For this review, take the finished solid that the model builds, in its own axes (mm). Face numbers are marked on the shaded views. Coordinates: 2 decimals unless noted, no trailing zeros. Loops run counter-clockwise (first coordinate to the right, second up) from the corner with the lowest first, then second, coordinate; pieces in that order, holes last. Notation, with made-up numbers: (54.5, 2.25) - (78.5, 2.25) arc R23 cw to (78.5, 27.25) - close; hole circle Ø8 at (82, -2). An arc over 180 degrees is marked (long way). Answer as a JSON object with one key per item and string values. Group by question number.
Item 1: We need section A-A (z = 5.25). Give the boundary of the cut face in (x, y).
Item 2: Mouldability with a two-part tool opening along X and no side actions: class the marked faces 1, 2 and 3 as released by +X, released by -X, zero draft, split by the parting line, or undercut.
Item 3: We need section C-C (y = -48). Give the boundary of the cut face in (x, z), then the cut area to 3 significant figures.
Item 4: We need section B-B (x = -4.85). Give the boundary of the cut face in (y, z).
Item 5: We need section D-D (z = 4.1). Give the boundary of the cut face in (x, y), then the cut area to 3 significant figures.
Item 6: To check wall thickness, follow line 1 (Y direction, x = -4.85, z = 3.2); line 2 (X direction, y = -56.25, z = 3.8); line 3 (X direction, y = -56.75, z = 3.3). State the ranges of each line that lie inside material, in increasing order.
Item 7: Clearance check with flat-ended pins moving along their axes: pin 1 (2 mm diameter, centred on y = -53, z = 4, fed in from +X); pin 2 (1.5 mm diameter, centred on y = -53.5, z = 4, fed in from -X). State where each tip first meets the part, or that it passes through.
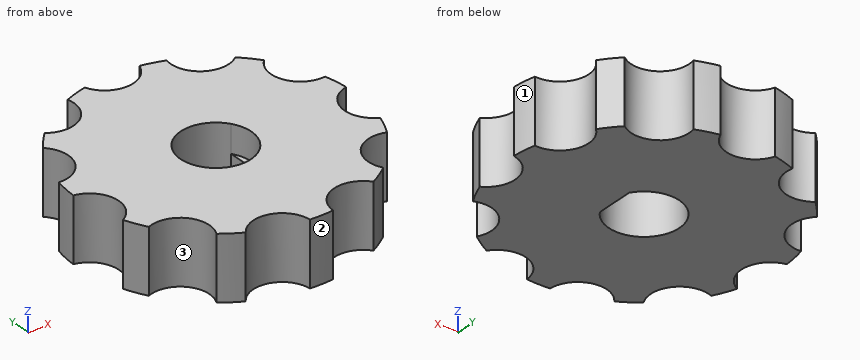
from build123d import *

# Parameters (mm, degrees)
SKETCH024_R           = 9.9166910254
PAD016_DEPTH          = 4.6
SKETCH025_R           = 2.1
POCKET004_DEPTH       = 61.4476740325
POLARPATTERN001_COUNT = 11
POCKET005_DEPTH       = 4.601
SKETCH037_R           = 2.55
POCKET012_DEPTH       = 2


with BuildPart() as part:
    # Sketch024 → Pad016 (new body)
    with BuildSketch(Plane.XY):
        Circle(SKETCH024_R)
    extrude(amount=PAD016_DEPTH)

    # Sketch025 (on Face3 of Pad016) → Pocket004 (cut, through all)
    with BuildSketch(Plane.XY.offset(4.6)):
        with Locations((0, 10.4166910254)):
            Circle(SKETCH025_R)
    pocket004 = extrude(amount=-POCKET004_DEPTH, mode=Mode.SUBTRACT)

    # PolarPattern001: Pocket004 ×11 about axis
    polarpattern001_axis = Axis((0, 0, 4.6), (0, 0, 1))
    for i in range(1, POLARPATTERN001_COUNT):
        add(pocket004.rotate(polarpattern001_axis, i * 360 / POLARPATTERN001_COUNT), mode=Mode.SUBTRACT)

    # Sketch026 (on Face4 of PolarPattern001) → Pocket005 (cut, through all)
    with BuildSketch(Plane.XY.offset(4.6)):
        with BuildLine():
            ThreePointArc((2.15, 1.3711309201), (-2.55, 0), (2.15, -1.3711309201))
            Line((2.15, -1.3711309201), (2.15, 1.3711309201))
        make_face()
    extrude(amount=-POCKET005_DEPTH, mode=Mode.SUBTRACT)

    # Sketch037 (on Face4 of Pocket005) → Pocket012 (cut)
    with BuildSketch(Plane.XY.offset(4.6)):
        Circle(SKETCH037_R)
    extrude(amount=-POCKET012_DEPTH, mode=Mode.SUBTRACT)


with BuildPart() as part_1:
    # Body004 placement: moved
    add(part.part.moved(Location((-4.85, -48.15, 2.2))))


solid = part_1.part
Check sheet entries:
{
 "1": {"outline": "(-14.75, -47.57) arc R2.1 cw to (-14.19, -51.49) arc R9.92 ccw to (-13.49, -53.02) arc R2.1 cw to (-10.9, -56.01) arc R9.92 ccw to (-9.49, -56.92) arc R2.1 cw to (-5.69, -58.03) arc R9.92 ccw to (-4.01, -58.03) arc R2.1 cw to (-0.21, -56.92) arc R9.92 ccw to (1.2, -56.01) arc R2.1 cw to (3.79, -53.02) arc R9.92 ccw to (4.49, -51.49) arc R2.1 cw to (5.05, -47.57) arc R9.92 ccw to (4.81, -45.91) arc R2.1 cw to (3.17, -42.31) arc R9.92 ccw to (2.07, -41.05) arc R2.1 cw to (-1.26, -38.91) arc R9.92 ccw to (-2.87, -38.43) arc R2.1 cw to (-6.83, -38.43) arc R9.92 ccw to (-8.44, -38.91) arc R2.1 cw to (-11.77, -41.05) arc R9.92 ccw to (-12.87, -42.31) arc R2.1 cw to (-14.51, -45.91) arc R9.92 ccw to start; hole circle Ø5.1 at (-4.85, -48.15)"},
 "2": {"face 1": "released by +X", "face 2": "split by the parting line", "face 3": "undercut"},
 "3": {"outline": "(-13.84, 2.2) - (-7.4, 2.2) - (-7.4, 6.8) - (-13.84, 6.8) - close; (-2.7, 2.2) - (4.14, 2.2) - (4.14, 6.8) - (-2.3, 6.8) - (-2.3, 4.8) - (-2.7, 4.8) - close", "area": "60.3 mm2"},
 "4": {"outline": "(-58.07, 2.2) - (-50.7, 2.2) - (-50.7, 6.8) - (-58.07, 6.8) - close; (-45.6, 2.2) - (-39.83, 2.2) - (-39.83, 6.8) - (-45.6, 6.8) - close"},
 "5": {"outline": "(-14.75, -47.57) arc R2.1 cw to (-14.19, -51.49) arc R9.92 ccw to (-13.49, -53.02) arc R2.1 cw to (-10.9, -56.01) arc R9.92 ccw to (-9.49, -56.92) arc R2.1 cw to (-5.69, -58.03) arc R9.92 ccw to (-4.01, -58.03) arc R2.1 cw to (-0.21, -56.92) arc R9.92 ccw to (1.2, -56.01) arc R2.1 cw to (3.79, -53.02) arc R9.92 ccw to (4.49, -51.49) arc R2.1 cw to (5.05, -47.57) arc R9.92 ccw to (4.81, -45.91) arc R2.1 cw to (3.17, -42.31) arc R9.92 ccw to (2.07, -41.05) arc R2.1 cw to (-1.26, -38.91) arc R9.92 ccw to (-2.87, -38.43) arc R2.1 cw to (-6.83, -38.43) arc R9.92 ccw to (-8.44, -38.91) arc R2.1 cw to (-11.77, -41.05) arc R9.92 ccw to (-12.87, -42.31) arc R2.1 cw to (-14.51, -45.91) arc R9.92 ccw to start; hole (-2.7, -49.52) - (-2.7, -46.78) arc R2.55 ccw (long way) to start", "area": "239 mm2"},
 "6": {"line 1": "y = -58.07 to -50.7, -45.6 to -39.83", "line 2": "x = -10.57 to -8.69, -6.88 to -2.82, -1.01 to 0.87", "line 3": "x = -9.79 to -9.35, -6.21 to -3.49, -0.35 to 0.09"},
 "7": {"pin 1": "stops at x = 4.29", "pin 2": "stops at x = -13.64"}
}
